Could you check a few things on this model? Use its own coordinates, in mm. Face numbers are marked on the shaded views. A direction names the side the tool comes from. Round coordinates to 2 decimals unless told otherwise and drop trailing zeros. Loops run counter-clockwise (first coordinate to the right, second up) from the corner with the lowest first, then second, coordinate; pieces in that order, holes last. Notation, with made-up numbers: (39, -7.5) -> (47, -7.5) arc R15 cw to (47, 21.5) -> close; hole circle Ø7 at (80, 46). An arc over 180 degrees is marked (long way). Put each result on its own line as item: value. Start each with the question number.
1. Imagine slicing it at A-A, the plane z = 5. Please give me the cut outline in (x, y), and give its area (3 significant figures).
2. I'm going to push flat-ended pins straight in: P1, Ø2.5, axis at x = -2, z = 3.5, coming from the +Y side; P2, Ø1.5, axis at y = 0, z = 6.5, coming from the +X side; P3, Ø2, axis at x = -11, y = -2, coming from the -Z side; P4, Ø1, axis at x = -14.5, z = 3, coming from the -Y side. Where does each tip first touch, or does it pass through?
3. Imagine slicing it at C-C, the plane z = 3.25. Please give me the cut outline in (x, y), and give its area (3 significant figures).
4. Imagine slicing it at D-D, the plane y = 0.15. Please give me the cut outline in (x, z), and give its area (3 significant figures).
5. Which directions (+Z, -Z, +X, -X, +Y, -Y) give clear straight access to the entire face, cutting with the end or side of a thin tool? Please do the marked faces 4 and 5.
6. Imagine slicing it at B-B, the plane y = -2. Please give me the cut outline in (x, z), and give its area (3 significant figures).
7. I need wall thicknesses on line 1 (X direction, y = -1.3, z = 5); line 2 (X direction, y = -1.75, z = 5); line 3 (Y direction, x = -15, z = 8.75). Which ranges of each line are inside material? Lowest first, please. Write a range as [from, to].
8. If we mould it in two halves opening along X, with no side actions, what happens to the marked faces 1, 2 and 3? For each: pulls with the +X half, pulls with the -X half, needs draft (parallel to the pull), parting line crosses it, or undercut.
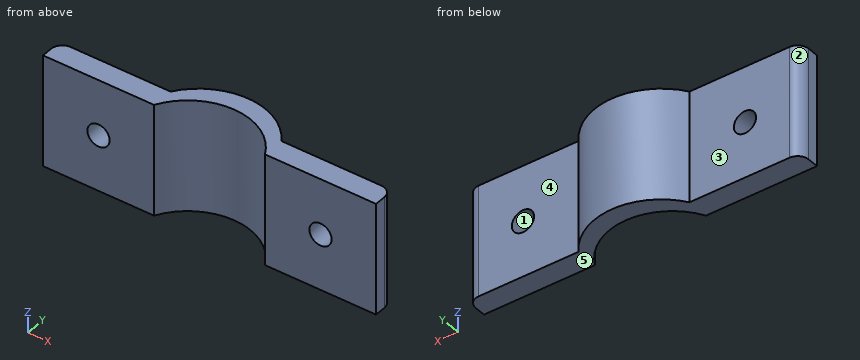
```python
from build123d import *

# Parameters (mm, degrees)
BOSS_EXTRUDE1_DEPTH = 10
SKETCH2_R           = 1
CUT_EXTRUDE1_DEPTH  = 10
FILLET1_R           = 1


with BuildPart() as part:
    # Sketch1 → Boss-Extrude1 (new body)
    with BuildSketch(Plane.XY):
        with BuildLine():
            Line((-24.705882353, -2.573529412), (-14.705882353, -2.573529412))
            ThreePointArc((-14.705882353, -2.573529412), (-9.705882353, 0.434570501), (-4.705882353, -2.573529412))
            Line((-4.705882353, -2.573529412), (5.294117647, -2.573529412))
            Line((5.294117647, -2.573529412), (5.294117647, -0.573529412))
            Line((5.294117647, -0.573529412), (-4.705882353, -0.573529412))
            ThreePointArc((-4.705882353, -0.573529412), (-9.705882353, 2.106978403), (-14.705882353, -0.573529412))
            Line((-14.705882353, -0.573529412), (-24.705882353, -0.573529412))
            Line((-24.705882353, -0.573529412), (-24.705882353, -2.573529412))
        make_face()
    extrude(amount=BOSS_EXTRUDE1_DEPTH)

    # Sketch2 → Cut-Extrude1 (cut)
    with BuildSketch(Plane(origin=(0, -0.573529412, 0), x_dir=(1, 0, 0), z_dir=(0, 1, 0))):
        with Locations(Location((0.294117647, -5, 0), (0, 0, 270))):
            Circle(SKETCH2_R)
        with Locations(Location((-19.705882353, -5, 0), (0, 0, 270))):
            Circle(SKETCH2_R)
    extrude(amount=-CUT_EXTRUDE1_DEPTH, mode=Mode.SUBTRACT)

    # Fillet1
    fillet1_edges = [part.edges().sort_by_distance(p)[0] for p in [
        (-24.705882353, -0.573529412, 5),
        (5.294117647, -0.573529412, 5),
    ]]
    fillet(fillet1_edges, radius=FILLET1_R)


solid = part.part
```
Entries:
1. outline: (-24.71, -2.57) -> (-20.71, -2.57) -> (-20.71, -0.57) -> (-23.71, -0.57) arc R1 ccw to (-24.71, -1.57) -> close; (-18.71, -2.57) -> (-14.71, -2.57) arc R5.66 cw to (-4.71, -2.57) -> (-0.71, -2.57) -> (-0.71, -0.57) -> (-4.71, -0.57) arc R6 ccw to (-14.71, -0.57) -> (-18.71, -0.57) -> close; (1.29, -2.57) -> (5.29, -2.57) -> (5.29, -1.57) arc R1 ccw to (4.29, -0.57) -> (1.29, -0.57) -> close
1. area: 49.0 mm^2
2. P1: y = -0.57
2. P2: x = 4.86
2. P3: through
2. P4: y = -2.57
3. outline: (-24.71, -2.57) -> (-14.71, -2.57) arc R5.66 cw to (-4.71, -2.57) -> (5.29, -2.57) -> (5.29, -1.57) arc R1 ccw to (4.29, -0.57) -> (-4.71, -0.57) arc R6 ccw to (-14.71, -0.57) -> (-23.71, -0.57) arc R1 ccw to (-24.71, -1.57) -> close
3. area: 57.0 mm^2
4. outline: (-14.14, 0) -> (-11.48, 0) -> (-11.48, 10) -> (-14.14, 10) -> close; (-7.93, 0) -> (-5.27, 0) -> (-5.27, 10) -> (-7.93, 10) -> close
4. area: 53.3 mm^2
5. face 4: +Z, -Z, +X, +Y
5. face 5: -Z, +X, -X, +Y, -Y
6. outline: (-24.71, 0) -> (-14.36, 0) -> (-14.36, 10) -> (-24.71, 10) -> close; (-5.06, 0) -> (5.29, 0) -> (5.29, 10) -> (-5.06, 10) -> close; hole circle Ø2 at (-19.71, 5); hole circle Ø2 at (0.29, 5)
6. area: 201 mm^2
7. line 1: [-24.67, -20.71], [-18.71, -13.78], [-5.63, -0.71], [1.29, 5.26]
7. line 2: [-24.71, -20.71], [-18.71, -14.17], [-5.24, -0.71], [1.29, 5.29]
7. line 3: [-2.57, -0.57]
8. face 1: undercut
8. face 2: pulls with the -X half
8. face 3: needs draft
